Model file for the job. Use its own axes, mm. Round coordinates to 2 decimals unless told otherwise and drop trailing zeros. Order: outer loops, then holes, each group sorted by start corner. A loop starts at its lowest first (then second) coordinate and runs counter-clockwise, first axis right, second up. Notation, with made-up numbers: (15, 5.25) -> (57, 5.25) arc R31 ccw to (57, 33.25) -> close; hole circle Ø10 at (2.5, 29.25). An arc over 180 degrees is marked (long way). Put each result on its own line as item: value. Start each with the question number.
Q1. Cut at C-C, the plane z = 3.5. State how many separate pieces and enclosed holes the cut face has, and give its area (3 significant figures).
Q2. Flat gauge pins, fed straight in: P1, Ø3, axis at x = 12.7, y = -95.25, coming from the -Z side; P2, Ø6.5, axis at x = 19.05, y = -41.275, coming from the -Z side. Where does each tip first touch, or does it go through?
Q3. Cut at B-B, the plane y = -69.85. List the corners of the cut face in (x, z) (3 decimals).
Q4. Cut at D-D, the plane x = -19.05. List the corners of the cut face in (y, z), and give its area (3 significant figures).
Q5. Cut at A-A, the plane x = 0. List the corners of the cut face in (y, z), and give its area (3 significant figures).
Q6. Probe L1, parallel to X at y = 12.7, z = 3.75 (3 decimals); L2, parallel to Y at x = -19.05, z = 3.5; L3, parallel to X at y = -95.25, z = 2.75 (3 decimals). List the from-to ranges inside material, lowest first.
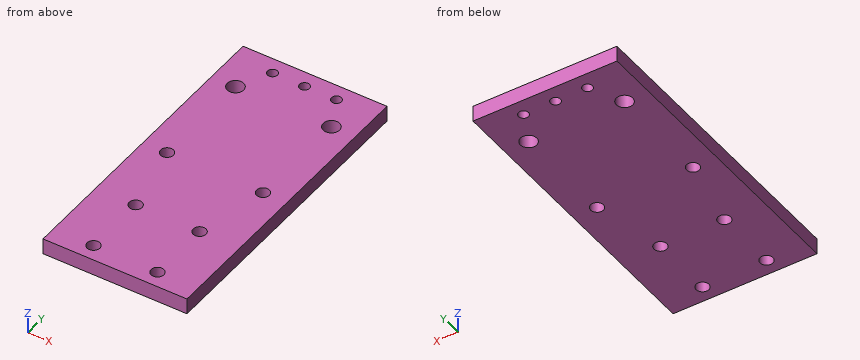
Autodesk Inventor part; units mm, degrees
ref_plane "YZ Plane" through (0, 0, 0) normal (1, 0, 0) x (0, 1, 0)
ref_plane "XZ Plane" through (0, 0, 0) normal (0, 1, 0) x (-1, 0, 0)
ref_plane "XY Plane" through (0, 0, 0) normal (0, 0, 1) x (1, 0, 0)
sketch "Sketch1" plane through (0, 0, 0) normal (0, 0, 1) x (1, 0, 0)
  line L0 (-19.05, 0) -> (19.05, 0) construction
  circle A0 centre (-19.05, 0) radius 3.2639
  circle A1 centre (19.05, 0) radius 3.2639
  line L1 (-28.575, 19.5947) -> (-28.575, -101.6)
  line L2 (-28.575, -101.6) -> (28.575, -101.6)
  line L3 (28.575, -101.6) -> (28.575, 19.5947)
  line L4 (-26.7151, 24.0849) -> (-4.4901, 46.3099)
  line L5 (4.4901, 46.3099) -> (26.7151, 24.0849)
  arc A2 (4.4901, 46.3099) -> (-4.4901, 46.3099) centre (0, 41.8197) ccw
  arc A3 (-26.7151, 24.0849) -> (-28.575, 19.5947) centre (-22.225, 19.5947) ccw
  arc A4 (28.575, 19.5947) -> (26.7151, 24.0849) centre (22.225, 19.5947) ccw
  line L6 (-28.575, 19.05) -> (28.575, 19.05)
  line L7 (-12.7, 12.7) -> (12.7, 12.7) construction
  line L8 (-12.7, -69.85) -> (12.7, -69.85) construction
  point P0 (0, 0)
  point P1 (0, 0)
  point P2 (0, 50.8)
  point P3 (28.575, 22.225)
  point P4 (-28.575, 22.225)
  point P5 (0, -101.6)
  point P6 (0, 12.7)
  point P7 (0, 12.7)
  point P8 (-12.7, -95.25)
  point P9 (12.7, -95.25)
  point P10 (0, -69.85)
  dimension "d0" = 6.5278
  dimension "d1" = 38.1
  dimension "d4" = 101.6
  dimension "d17" = 152.4
  dimension "d18" = 57.15
  dimension "d19" = 6.35
  dimension "d20" = 120.65
  dimension "d21" = 25.4
  dimension "d29" = 6.35
  dimension "d32" = 25.4
  dimension "d33" = 25.4
  dimension "d34" = 6.35
  dimension "d42" = 12.7
  dimension "d43" = 19.05
extrude "Extrusion1" add sketch "Sketch1" along normal blind 6.35 contours L6 L3 L2 L1
sketch "Sketch2" plane through (0, 0, 6.35) normal (0, 0, 1) x (1, 0, 0)
  line L0 (-19.05, -41.275) -> (19.05, -41.275) construction
  line L1 (-28.575, -101.6) -> (28.575, -101.6)
  point P0 (0, 0)
  point P1 (0, -41.275)
  dimension "d8" = 38.1
  dimension "d9" = 60.325
hole "Hole1" at (-19.05, -41.275, 6.35) at (19.05, -41.275, 6.35) direction (0, 0, -1) diameter 5.1054 end through all
hole "Hole2" at (-12.7, 12.7, 0) at (0, 12.7, 0) at (12.7, 12.7, 0) direction (0, 0, 1) diameter 3.9624 end through all
hole "Hole3" at (-12.7, -69.85, 0) at (12.7, -69.85, 0) at (-12.7, -95.25, 0) at (12.7, -95.25, 0) direction (0, 0, 1) diameter 5.1054 end through all
properties part number "CL7-005" material "Aluminum 6061"
Ans:
1. separate pieces: 1
1. enclosed holes: 11
1. area: 6,670 mm^2
2. P1: passes through
2. P2: stops at z = 0
3. outline: (-28.575, 0) -> (-15.253, 0) -> (-15.253, 6.35) -> (-28.575, 6.35) -> close; (-10.147, 0) -> (10.147, 0) -> (10.147, 6.35) -> (-10.147, 6.35) -> close; (15.253, 0) -> (28.575, 0) -> (28.575, 6.35) -> (15.253, 6.35) -> close
4. outline: (-101.6, 0) -> (-43.83, 0) -> (-43.83, 6.35) -> (-101.6, 6.35) -> close; (-38.72, 0) -> (-3.26, 0) -> (-3.26, 6.35) -> (-38.72, 6.35) -> close; (3.26, 0) -> (19.05, 0) -> (19.05, 6.35) -> (3.26, 6.35) -> close
4. area: 692 mm^2
5. outline: (-101.6, 0) -> (10.72, 0) -> (10.72, 6.35) -> (-101.6, 6.35) -> close; (14.68, 0) -> (19.05, 0) -> (19.05, 6.35) -> (14.68, 6.35) -> close
5. area: 741 mm^2
6. L1: x = -28.575 to -14.681, -10.719 to -1.981, 1.981 to 10.719, 14.681 to 28.575
6. L2: y = -101.6 to -43.83, -38.72 to -3.26, 3.26 to 19.05
6. L3: x = -28.575 to -15.253, -10.147 to 10.147, 15.253 to 28.575
